```python
from build123d import *

# Parameters (mm, degrees)
SKETCH1_W           = 26.6
SKETCH1_H           = 25
BOSS_EXTRUDE1_DEPTH = 2
SKETCH2_W           = 26.6
SKETCH2_H           = 2
BOSS_EXTRUDE2_DEPTH = 13
SKETCH3_W           = 4.4
SKETCH3_H           = 6.7
CUT_EXTRUDE1_DEPTH  = 3
FILLET1_R           = 2
SKETCH4_R           = 4
CUT_EXTRUDE2_DEPTH  = 3


with BuildPart() as part:
    # Sketch1 → Boss-Extrude1 (new body)
    with BuildSketch(Plane(origin=(0, 0, 0), x_dir=(1, 0, 0), z_dir=(0, 1, 0))):
        Rectangle(SKETCH1_W, SKETCH1_H)
    extrude(amount=BOSS_EXTRUDE1_DEPTH)

    # Sketch2 → Boss-Extrude2 (add)
    with BuildSketch(Plane(origin=(0, 2, 0), x_dir=(1, 0, 0), z_dir=(0, 1, 0))):
        with Locations((0, -11.5)):
            Rectangle(SKETCH2_W, SKETCH2_H)
    extrude(amount=BOSS_EXTRUDE2_DEPTH)

    # Sketch3 → Cut-Extrude1 (cut, through all)
    with BuildSketch(Plane(origin=(0, 0, 10.5), x_dir=(-1, 0, 0), z_dir=(0, 0, -1))):
        with Locations((-8, 10)):
            Rectangle(SKETCH3_W, SKETCH3_H)
        with Locations((8, 10)):
            Rectangle(SKETCH3_W, SKETCH3_H)
    extrude(amount=-CUT_EXTRUDE1_DEPTH, mode=Mode.SUBTRACT)

    # Fillet1
    fillet1_edges = [part.edges().sort_by_distance(p)[0] for p in [
        (-13.3, 1, -12.5),
        (13.3, 1, -12.5),
        (5.8, 6.65, 11.5),
        (10.2, 6.65, 11.5),
        (-10.2, 6.65, 11.5),
        (-5.8, 6.65, 11.5),
        (-10.2, 13.35, 11.5),
        (-5.8, 13.35, 11.5),
        (5.8, 13.35, 11.5),
        (10.2, 13.35, 11.5),
        (13.3, 15, 11.5),
        (-13.3, 15, 11.5),
    ]]
    fillet(fillet1_edges, radius=FILLET1_R)

    # Sketch4 → Cut-Extrude2 (cut, through all)
    with BuildSketch(Plane(origin=(0, 2, 0), x_dir=(1, 0, 0), z_dir=(0, 1, 0))):
        with Locations((0, 3.5)):
            Circle(SKETCH4_R)
    extrude(amount=-CUT_EXTRUDE2_DEPTH, mode=Mode.SUBTRACT)


solid = part.part
```
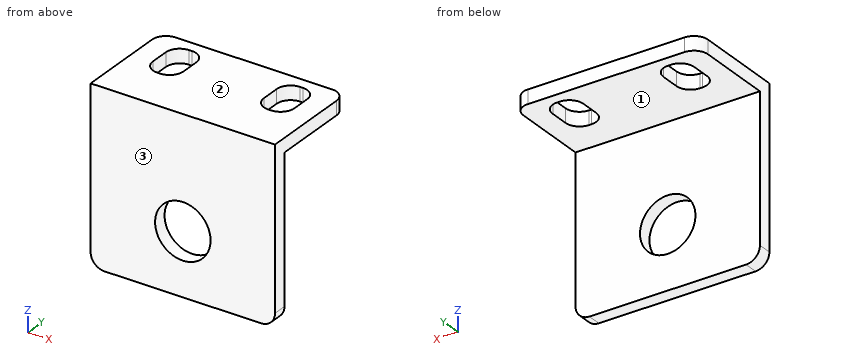
The listing builds one solid part. Answer for the finished solid, in the listing's coordinates (mm). Face numbers are marked on the shaded views. Coordinates: 2 decimals unless noted, no trailing zeros. Order: outer loops, then holes, each group sorted by start corner. A loop starts at its lowest first (then second) coordinate and runs counter-clockwise, first axis right, second up. Notation, with made-up numbers: M 56.25,6.25 L 68.25,6.25 A23 ccw 68.25,23.25 Z; hole C -21.75,85 d11. An arc over 180 degrees is marked long. Answer as a JSON object with one key per item and string values. Group by question number.
1. Section C-C on y = 8.25 is taken. Write down the section's boundary in (x, z), then the cut area to 3 significant figures.
2. Section B-B on z = -3.5 is taken. Write down the section's boundary in (x, y), then the cut area to 3 significant figures.
3. Section A-A on x = 0 is taken. Write down the section's boundary in (y, z), then the cut area to 3 significant figures.
4. A flat-ended cylindrical pin translates along its axis: P1, Ø6, axis at x = 3.5, z = 2, coming from the -Y side. Find the tip coordinate at first contact, or state that the pin passes through.
5. Determine the mould class of the marked faces 1, 2 and 3 for opening direction Z: released by +Z, released by -Z, zero draft, split by the parting line, or undercut.
6. Straight lines are drawn through the part: line 1 (Z direction, x = 0, y = 1.35); line 2 (X direction, y = 0.8, z = -3.5); line 3 (Y direction, x = -5.25, z = -0.25). For each, find the intervals that lie inside material, in ascending order.
7. Section D-D on x = 3 is taken. Write down the section's boundary in (y, z), then the cut area to 3 significant figures.
Values follow:
{
 "1": {"outline": "M -13.3,10.5 L -10.16,10.5 L -10.16,12.5 L -13.3,12.5 Z; M -5.84,10.5 L 5.84,10.5 L 5.84,12.5 L -5.84,12.5 Z; M 10.16,10.5 L 13.3,10.5 L 13.3,12.5 L 10.16,12.5 Z", "area": "35.9 mm2"},
 "2": {"outline": "M -13.3,0 L -4,0 L -4,2 L -13.3,2 Z; M 4,0 L 13.3,0 L 13.3,2 L 4,2 Z", "area": "37.2 mm2"},
 "3": {"outline": "M 0,-12.5 L 2,-12.5 L 2,-7.5 L 0,-7.5 Z; M 0,0.5 L 2,0.5 L 2,10.5 L 15,10.5 L 15,12.5 L 0,12.5 Z", "area": "60.0 mm2"},
 "4": {"P1": "y = 0"},
 "5": {"face 1": "released by -Z", "face 2": "released by +Z", "face 3": "zero draft"},
 "6": {"line 1": "-12.5 to -7.5, 0.5 to 12.5", "line 2": "-13.3 to -4, 4 to 13.3", "line 3": "0 to 2"},
 "7": {"outline": "M 0,-12.5 L 2,-12.5 L 2,-6.15 L 0,-6.15 Z; M 0,-0.85 L 2,-0.85 L 2,10.5 L 15,10.5 L 15,12.5 L 0,12.5 Z", "area": "65.4 mm2"}
}
